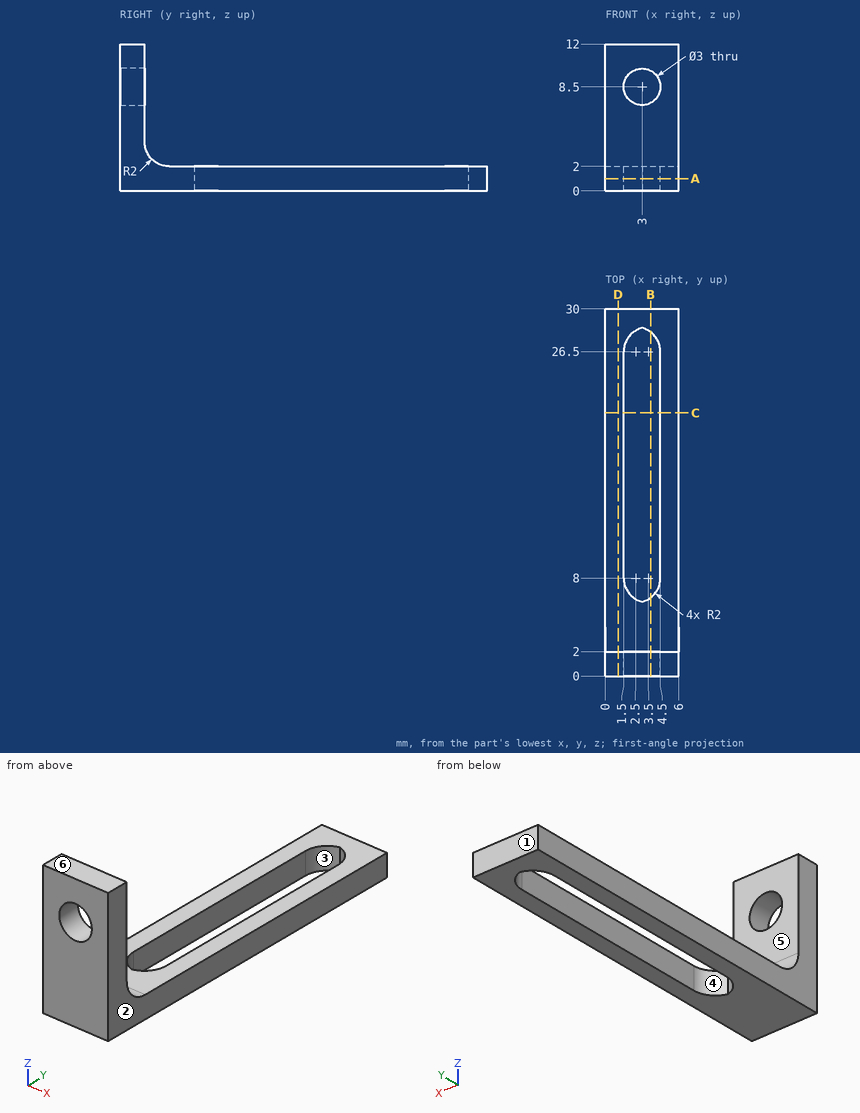
Input: dimensioned drawing with shaded views. Units: mm. Origin: part minimum x, y, z. A direction names the side the tool comes from. Give positions to 0.01 mm unless a question says otherwise; leave off trailing zeros. Write each loop counter-clockwise with the first axis right and the second up, starting at its lowest first coordinate (ties: lowest second). Pieces come first, ordered by that corner, then holes.
1. Section query A-A, the plane z = 1. Return loops of the section in (x, y), then the cut area to 3 significant figures.
2. Line query: probe 1 along X at (y, z) = (1.45, 8.5); probe 2 along Y at (x, z) = (3.55, 5); probe 3 along Y at (x, z) = (5.7, 3.25). Output: solid intervals per line, ascending.
3. Section query D-D, the plane x = 1.05. Return loops of the section in (y, z), then the cut area to 3 significant figures.
4. Draft query along X for the marked faces 1, 2 and 3. Return one class per face: released by +X, released by -X, zero draft, split by the parting line, or undercut.
5. Pin query (flat end, axial travel): P1, Ø1.5, axis at x = 4.5, y = 20, coming from the +Z side; P2, Ø2, axis at x = 2, z = 10.5, coming from the +Y side; P3, Ø1, axis at x = 0.5, y = 4, coming from the +Z side. Return the tip coordinate at first contact, or that it passes through.
6. Section query C-C, the plane y = 21.5. Return loops of the section in (x, z).
7. Reachability of the marked faces 4, 5 and 6 from +Z, -Z, +X, -X, +Y, -Y: full face, straight path, thin tool, end or side. Return the list, or none.
8. Section query B-B, the plane x = 3.7. Return loops of the section in (y, z), then the cut area to 3 significant figures.
Computed:
1. outline: (0, 0) - (6, 0) - (6, 30) - (0, 30) - close; hole (1.5, 8) arc R2 ccw to (3, 6.06) arc R2 ccw to (4.5, 8) - (4.5, 26.5) arc R2 ccw to (3, 28.44) arc R2 ccw to (1.5, 26.5) - close
1. area: 116 mm2
2. probe 1: x = 0 to 1.5, 4.5 to 6
2. probe 2: y = 0 to 2
2. probe 3: y = 0 to 2.15
3. outline: (0, 0) - (30, 0) - (30, 2) - (4, 2) arc R2 cw to (2, 4) - (2, 12) - (0, 12) - close
3. area: 80.9 mm2
4. face 1: zero draft
4. face 2: released by +X
4. face 3: undercut
5. P1: stops at z = 2
5. P2: stops at y = 2
5. P3: stops at z = 2.06
6. outline: (0, 0) - (1.5, 0) - (1.5, 2) - (0, 2) - close; (4.5, 0) - (6, 0) - (6, 2) - (4.5, 2) - close
7. face 4: +Z, -Z
7. face 5: +Z, +X, -X, +Y
7. face 6: +Z, +X, -X, +Y, -Y
8. outline: (0, 0) - (6.4, 0) - (6.4, 2) - (4, 2) arc R2 cw to (2, 4) - (2, 7.17) - (0, 7.17) - close; (0, 9.83) - (2, 9.83) - (2, 12) - (0, 12) - close; (28.1, 0) - (30, 0) - (30, 2) - (28.1, 2) - close
8. area: 32.2 mm2
